The listing builds one solid part. Answer for the finished solid, in the listing's coordinates (mm). A direction names the side the tool comes from. Give positions to 0.01 mm unless a question says otherwise; leave off trailing zeros. Order: outer loops, then holes, each group sorted by start corner. A loop starts at its lowest first (then second) coordinate and runs counter-clockwise, first axis right, second up. Notation, with made-up numbers: (55, 25) - (109, 25) arc R16 cw to (109, 55) - close; hole circle Ø2 at (69, 58.5). An arc over 180 degrees is marked (long way). Answer in a Markdown table with one row per item.
from build123d import *

# Parameters (mm, degrees)
F1_DEPTH = 30
F2_W     = 43.2
F2_H     = 18.8
F3_DEPTH = 15.3


with BuildPart() as f1:
    # F0 (on Top) → F1 (new body)
    with BuildSketch(Plane.XY):
        with BuildLine():
            Line((22.0444222056, -29.4440398328), (-0.0914469621, -29.4440398328))
            Line((-0.0914469621, -29.4440398328), (-0.0914469621, -49.2588512566))
            Line((-0.0914469621, -49.2588512566), (25.9435530379, -75.2938512566))
            Line((25.9435530379, -75.2938512566), (44.6278690687, -93.9781672875))
            ThreePointArc((44.6278690687, -93.9781672875), (57.8553211437, -86.5395948889), (69.8723409305, -77.2719585577))
            Line((69.8723409305, -77.2719585577), (22.0444222056, -29.4440398328))
        make_face()
        with BuildLine():
            Line((-22.2273161299, -29.4440398328), (-70.0552348548, -77.2719585577))
            ThreePointArc((-70.0552348548, -77.2719585577), (-58.038215068, -86.5395948889), (-44.810762993, -93.9781672875))
            Line((-44.810762993, -93.9781672875), (-26.1264469621, -75.2938512566))
            Line((-26.1264469621, -75.2938512566), (-0.0914469621, -49.2588512566))
            Line((-0.0914469621, -49.2588512566), (-0.0914469621, -29.4440398328))
            Line((-0.0914469621, -29.4440398328), (-22.2273161299, -29.4440398328))
        make_face()
        Polygon((-0.0914469621, -49.2588512566), (-26.1264469621, -75.2938512566), (-0.0914469621, -75.2938512566), align=None)
        Polygon((-0.0914469621, -49.2588512566), (-0.0914469621, -75.2938512566), (25.9435530379, -75.2938512566), align=None)
    extrude(amount=F1_DEPTH)

    # F2 (on face) → F3 (cut)
    with BuildSketch(Plane.XZ.offset(75.2938512566)):
        with Locations((0, 14.9999954)):
            Rectangle(F2_W, F2_H)
    extrude(amount=-F3_DEPTH, mode=Mode.SUBTRACT)


solid = f1.part
Item 1: Determine the mould class of faces 4 (the face through (-1, -61, 30)), 5 (the face through (0, -68, 24.4)), 6 (the face through (-21.6, -68, 15)), 7 (the face through (57.678, -86.657, 14.79)) for opening direction Z: pulls with the +Z half, pulls with the -Z half, needs draft (parallel to the pull), parting line crosses it, or undercut.
Answer block:
| item | result |
|---|---|
| face 4 | pulls with the +Z half |
| face 5 | undercut |
| face 6 | undercut |
| face 7 | needs draft |
Item 2: Which of the six approach directions +Z, -Z, +X, -X, +Y, -Y give full straight-line access (tool end or side, diameter ignored) to faces 1 (the face through (-45.806, -53.023, 14.79)), 2 (the face through (21.6, -68, 15)), 3 (the face through (0, -75.294, 5))?
Answer block:
| item | result |
|---|---|
| face 1 | +Z, -Z, -X, +Y |
| face 2 | -Y |
| face 3 | +Z, -Z, -Y |
Item 3: Find section C-C on x = -8.5. Write down the section's boundary in (y, z).
Answer block:
| item | result |
|---|---|
| outline | (-75.29, 0) - (-29.44, 0) - (-29.44, 30) - (-75.29, 30) - (-75.29, 24.4) - (-59.99, 24.4) - (-59.99, 5.6) - (-75.29, 5.6) - close |
Item 4: Find section B-B on y = -74. Write down the section's boundary in (x, z).
Answer block:
| item | result |
|---|---|
| outline | (-66.78, 0) - (66.6, 0) - (66.6, 30) - (-66.78, 30) - close; hole (-21.6, 5.6) - (21.6, 5.6) - (21.6, 24.4) - (-21.6, 24.4) - close |
Item 5: Each of these flat-tipped pins is pushed along its axis until it touches: P1, Ø1, axis at y = -39, z = 5.5, coming from the +X side; P2, Ø1.5, axis at x = -52.5, z = 24.5, coming from the -Y side; P3, Ø12, axis at y = -64, z = 12.5, coming from the +X side. Where does it stop, or does it pass through?
Answer block:
| item | result |
|---|---|
| P1 | x = 32.1 |
| P2 | y = -90.39 |
| P3 | x = 62.6 |
Item 6: Consider line 1 (Z direction, x = -2.5, y = -72.5); line 2 (Y direction, x = -20.5, z = 18); line 3 (Y direction, x = 12.5, z = 2.5). Determine where each line is inside the solid, lowest interval first.
Answer block:
| item | result |
|---|---|
| line 1 | 0 to 5.6, 24.4 to 30 |
| line 2 | -59.99 to -29.44 |
| line 3 | -75.29 to -29.44 |
Item 7: Find section A-A on z = 20.5. Write down the section's boundary in (x, y).
Answer block:
| item | result |
|---|---|
| outline | (-70.06, -77.27) arc R105 ccw to (-44.81, -93.98) - (-26.13, -75.29) - (-21.6, -75.29) - (-21.6, -59.99) - (21.6, -59.99) - (21.6, -75.29) - (25.94, -75.29) - (44.63, -93.98) arc R105 ccw to (69.87, -77.27) - (22.04, -29.44) - (-22.23, -29.44) - close |
Item 8: Find section D-D on y = -82.5. Write down the section's boundary in (x, z).
Answer block:
| item | result |
|---|---|
| outline | (-63.72, 0) - (-33.33, 0) - (-33.33, 30) - (-63.72, 30) - close; (33.15, 0) - (63.54, 0) - (63.54, 30) - (33.15, 30) - close |
